```python
from build123d import *

# Parameters (mm, degrees)
F0_W     = 63.5
F0_H     = 19.05
F1_DEPTH = 12.7
F2_R     = 3.81
F3_DEPTH = 12.7


# Not quite as in the source:
# - a feature names something its author has since deleted; it is built from what else it names


with BuildPart() as f1:
    # F0 (on Front) → F1 (new body, symmetric)
    with BuildSketch(Plane.XZ):
        with Locations((31.75, -9.525)):
            Rectangle(F0_W, F0_H)
    extrude(amount=F1_DEPTH, both=True)

    # F2 (on face) → F3 (cut)
    with BuildSketch(Plane.XY):
        with Locations((44.45, 0)):
            Circle(F2_R)
        with Locations((19.05, 0)):
            Circle(F2_R)
    extrude(amount=-F3_DEPTH, mode=Mode.SUBTRACT)


solid = f1.part
```
Geometry: final body of the model. Coordinates: model frame, mm. A direction names the side the tool comes from. Give positions to 0.01 mm unless a question says otherwise; leave off trailing zeros. Write each loop counter-clockwise with the first axis right and the second up, starting at its lowest first coordinate (ties: lowest second). Pieces come first, ordered by that corner, then holes.
1. Section query B-B, the plane y = 0. Return loops of the section in (x, z).
2. Draft query along Y for faces 3 (the flat face through (0, 0, -10)), 4 (the cylindrical face through (40.644, 0.168, -6.261)), 5 (the flat face through (44, 0, -12.7)), 6 (the flat face through (31, 12.7, -9)). Return one class per face: released by +Y, released by -Y, zero draft, split by the parting line, or undercut.
3. Reachability of faces 1 (the flat face through (31, -12.7, -9)), 2 (the flat face through (19, 0, -12.7)) from +Z, -Z, +X, -X, +Y, -Y: full face, straight path, thin tool, end or side. Return the list, or none.
4. Section query C-C, the plane x = 44.45. Return loops of the section in (y, z).
5. Line query: probe 1 along Y at (x, z) = (44.45, -10); probe 2 along X at (y, z) = (-3, -3.5); probe 3 along X at (y, z) = (2.75, -8). Output: solid intervals per line, ascending.
6. Section query A-A, the plane z = -6.5. Return loops of the section in (x, y), then the cut area to 3 significant figures.
Computed:
1. outline: (0, -19.05) - (63.5, -19.05) - (63.5, 0) - (48.26, 0) - (48.26, -12.7) - (40.64, -12.7) - (40.64, 0) - (22.86, 0) - (22.86, -12.7) - (15.24, -12.7) - (15.24, 0) - (0, 0) - close
2. face 3: zero draft
2. face 4: undercut
2. face 5: undercut
2. face 6: released by +Y
3. face 1: +Z, -Z, +X, -X, -Y
3. face 2: +Z
4. outline: (-12.7, -19.05) - (12.7, -19.05) - (12.7, 0) - (3.81, 0) - (3.81, -12.7) - (-3.81, -12.7) - (-3.81, 0) - (-12.7, 0) - close
5. probe 1: y = -12.7 to -3.81, 3.81 to 12.7
5. probe 2: x = 0 to 16.7, 21.4 to 42.1, 46.8 to 63.5
5. probe 3: x = 0 to 16.41, 21.69 to 41.81, 47.09 to 63.5
6. outline: (0, -12.7) - (63.5, -12.7) - (63.5, 12.7) - (0, 12.7) - close; hole circle Ø7.62 at (19.05, 0); hole circle Ø7.62 at (44.45, 0)
6. area: 1,520 mm2
